```python
from build123d import *

# Parameters (mm, degrees)
SKETCH086_R     = 5.75
PAD036_DEPTH    = 15
SKETCH087_R     = 39
PAD037_DEPTH    = 3
SKETCH090_R     = 39
SKETCH090_R_2   = 38
PAD040_DEPTH    = 10
POCKET042_DEPTH = 5
SKETCH092_R     = 2.5
POCKET043_DEPTH = 5
POCKET044_DEPTH = 4.5


with BuildPart() as part:
    # Sketch086 → Pad036 (new body)
    with BuildSketch(Plane.XZ):
        with Locations((52.5, -57.86)):
            Circle(SKETCH086_R)
    extrude(amount=PAD036_DEPTH)

    # Sketch087 (on Face2 of Pad036) → Pad037 (join)
    with BuildSketch(Plane(origin=(0, 0, 0), x_dir=(1, 0, 0), z_dir=(0, 1, 0))):
        with Locations((52.5, 57.86)):
            Circle(SKETCH087_R)
    extrude(amount=PAD037_DEPTH)

    # Sketch090 → Pad040 (join)
    with BuildSketch(Plane.XZ):
        with Locations((52.5, -57.86)):
            Circle(SKETCH090_R)
        with Locations((52.5, -57.86)):
            Circle(SKETCH090_R_2, mode=Mode.SUBTRACT)
    extrude(amount=PAD040_DEPTH)

    # Sketch091 (on Face6 of Pad040) → Pocket042 (cut)
    with BuildSketch(Plane.XZ):
        with BuildLine():
            ThreePointArc((35.9062672696, -50.8851857321), (52.5, -75.86), (69.0937327304, -50.8851857321))
            Line((69.0937327304, -50.8851857321), (59.439457, -50.8851857321))
            Line((59.439457, -50.8851857321), (59.439457, -56.9413398097))
            ThreePointArc((45.6135845341, -56.6041011066), (52.3293077717, -64.8579185593), (59.439457, -56.9413398097))
            Line((45.6135845341, -56.6041011066), (45.6135845341, -50.8851857321))
            Line((45.6135845341, -50.8851857321), (35.9062672696, -50.8851857321))
        make_face()
    extrude(amount=-POCKET042_DEPTH, mode=Mode.SUBTRACT)

    # Sketch092 (on Face3 of Pocket042) → Pocket043 (cut)
    with BuildSketch(Plane(origin=(0, 3, 0), x_dir=(1, 0, 0), z_dir=(0, 1, 0))):
        with Locations((17.9137178727, 57.86)):
            Circle(SKETCH092_R)
        with Locations((26.5848547865, 57.86)):
            Circle(SKETCH092_R)
        with Locations((52.5, 92.4462821273)):
            Circle(SKETCH092_R)
        with Locations((52.5, 83.7751452135)):
            Circle(SKETCH092_R)
        with Locations((78.4151452135, 57.86)):
            Circle(SKETCH092_R)
        with Locations((87.0862821273, 57.86)):
            Circle(SKETCH092_R)
        with Locations((52.5, 31.9448547865)):
            Circle(SKETCH092_R)
        with Locations((52.5, 23.2737178727)):
            Circle(SKETCH092_R)
    extrude(amount=-POCKET043_DEPTH, mode=Mode.SUBTRACT)

    # Sketch093 (on Face22 of Pocket043) → Pocket044 (cut)
    with BuildSketch(Plane.XZ.offset(15)):
        with BuildLine():
            ThreePointArc((49.0466730198, -57.0371799905), (52.5000100371, -61.41), (55.9533223273, -57.037160463))
            Line((55.5, -53.178869006), (55.9533223273, -57.037160463))
            Line((49.5, -53.178869006), (55.5, -53.178869006))
            Line((49.0466730198, -57.0371799905), (49.5, -53.178869006))
        make_face()
    extrude(amount=-POCKET044_DEPTH, mode=Mode.SUBTRACT)


with BuildPart() as part_1:
    # Body011 placement: moved
    add(part.part.moved(Location((0, 189, 0))))


solid = part_1.part
```
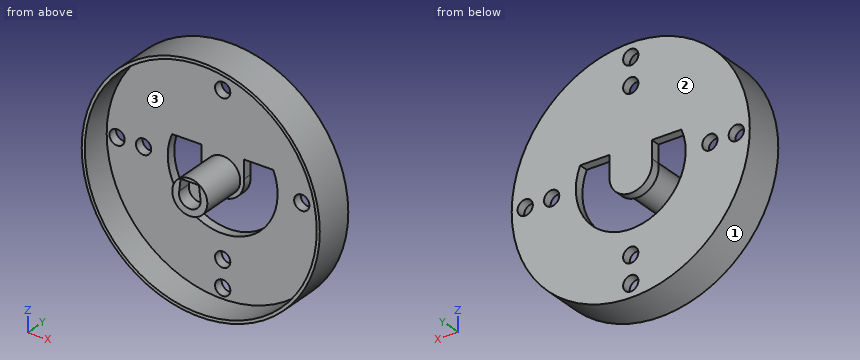
Work out the finished part from the listing and answer in its coordinate system (mm). Face numbers are marked on the shaded views. Give positions to 0.01 mm unless a question says otherwise; leave off trailing zeros. Loops run counter-clockwise (first coordinate to the right, second up) from the corner with the lowest first, then second, coordinate; pieces in that order, holes last. Notation, with made-up numbers: (-15, 23.5) - (44, 23.5) arc R19 ccw to (44, 38.5) - close; hole circle Ø4 at (60, 19.5). An arc over 180 degrees is marked (long way). One line per question, with ' | ' between items.
(1) The part is cut by section C-C (z = -74). Write down the section's boundary in (x, y), then the cut area to 3 significant figures.
Recorded:
outline: (17, 179) - (18.1, 179) - (18.1, 189) - (44.53, 189) - (44.53, 192) - (17, 192) - close; (60.47, 189) - (86.9, 189) - (86.9, 179) - (88, 179) - (88, 192) - (60.47, 192) - close | area: 187 mm²
(2) Straight lines are drawn through the part: probe 1 along Z at (x, y) = (52.5, 189.9); probe 2 along X at (y, z) = (185.25, -57.5); probe 3 along Z at (x, y) = (52.5, 183.5). For each, find the intervals that lie inside material, in ascending order.
Recorded:
probe 1: z = -96.86 to -94.95, -89.95 to -86.28, -81.28 to -75.86, -64.86 to -34.44, -29.44 to -25.77, -20.77 to -18.86 | probe 2: x = 13.5 to 14.5, 46.76 to 58.24, 90.5 to 91.5 | probe 3: z = -96.86 to -95.86, -63.61 to -52.11, -19.86 to -18.86
(3) The part is cut by section D-D (y = 188). Write down the section's boundary in (x, z), then the cut area to 3 significant figures.
Recorded:
outline: circle Ø78 at (52.5, -57.86); circle Ø11.5 at (52.5, -57.86); hole circle Ø76 at (52.5, -57.86) | area: 346 mm²
(4) Each of these flat-tipped pins is pushed along its axis until it touches: pin 1 Ø1 at (x, y) = (39, 185) entering from -Z; pin 2 Ø5 at (x, y) = (78.5, 178.5) entering from -Z; pin 3 Ø2 at (y, z) = (179.5, -78) entering from -X. Where does it stop, or does it pass through?
Recorded:
pin 1: stops at z = -94.63 | pin 2: stops at z = -88.95 | pin 3: stops at x = 18.52
(5) The mould has two halves that part along Z. Classify the marked faces 1, 2 and 3: +Z half, -Z half, draft (parallel to the pull), parting line (faces both ways), or undercut.
Recorded:
face 1: parting line | face 2: draft | face 3: undercut
(6) The part is cut by section A-A (y = 175). Write down the section's boundary in (x, z).
Recorded:
outline: circle Ø11.5 at (52.5, -57.86); hole (49.05, -57.04) arc R3.55 ccw (long way) to (55.95, -57.04) - (55.5, -53.18) - (49.5, -53.18) - close
(7) The part is cut by section B-B (x = 52.5). Count the separate pieces of the cut face and the enclosed holes in it, then the cut area to 3 significant figures.
Recorded:
separate pieces: 6 | enclosed holes: 0 | area: 296 mm²
